```python
from build123d import *

# Parameters (mm, degrees)
SKETCH1_W           = 197
SKETCH1_H           = 107
BOSS_EXTRUDE1_DEPTH = 50
SKETCH4_W           = 182
SKETCH4_H           = 45
CUT_EXTRUDE2_DEPTH  = 25
CUT_EXTRUDE3_DEPTH  = 164
CUT_EXTRUDE12_DEPTH = 164
CUT_EXTRUDE5_DEPTH  = 230.691096911
SKETCH9_R           = 8
CUT_EXTRUDE6_DEPTH  = 171
SKETCH10_R          = 10
CUT_EXTRUDE7_DEPTH  = 1.5
SKETCH11_R          = 4.8
CUT_EXTRUDE8_DEPTH  = 12.5
SKETCH12_R          = 6.5
CUT_EXTRUDE9_DEPTH  = 230.691096911
SKETCH13_R          = 3
CUT_EXTRUDE10_DEPTH = 26.5
SKETCH14_R          = 3
CUT_EXTRUDE11_DEPTH = 26.5
CUT_EXTRUDE14_DEPTH = 35
CUT_EXTRUDE15_DEPTH = 130


with BuildPart() as part:
    # Sketch1 → Boss-Extrude1 (new body)
    with BuildSketch(Plane(origin=(0, 0, 0), x_dir=(1, 0, 0), z_dir=(0, 1, 0))):
        with Locations((98.5, 53.5)):
            Rectangle(SKETCH1_W, SKETCH1_H)
    extrude(amount=BOSS_EXTRUDE1_DEPTH)

    # Sketch4 → Cut-Extrude2 (cut)
    with BuildSketch(Plane(origin=(0, 0, 0), x_dir=(1, 0, 0), z_dir=(0, 1, 0))):
        with Locations((98.5, 53.5)):
            Rectangle(SKETCH4_W, SKETCH4_H)
    extrude(amount=CUT_EXTRUDE2_DEPTH, mode=Mode.SUBTRACT)

    # Sketch5 → Cut-Extrude3 (cut)
    with BuildSketch(Plane(origin=(197, 0, 0), x_dir=(0, 0, -1), z_dir=(1, 0, 0))):
        Polygon((58.5, 50), (107, 44.216725137), (107, 50), align=None)
    extrude(amount=-CUT_EXTRUDE3_DEPTH, mode=Mode.SUBTRACT)

    # Sketch18 → Cut-Extrude12 (cut)
    with BuildSketch(Plane(origin=(197, 0, 0), x_dir=(0, 0, -1), z_dir=(1, 0, 0))):
        Polygon((0, 44.216725137), (0, 50), (48.5, 50), align=None)
    extrude(amount=-CUT_EXTRUDE12_DEPTH, mode=Mode.SUBTRACT)

    # Sketch7 → Cut-Extrude5 (cut, through all)
    with BuildSketch(Plane(origin=(0, 0, 0), x_dir=(0, 0, -1), z_dir=(1, 0, 0))):
        Polygon((107, 50), (107, 45), (82.505102572, 50), align=None)
        Polygon((0, 45), (0, 50), (24.494897428, 50), align=None)
    extrude(amount=CUT_EXTRUDE5_DEPTH, mode=Mode.SUBTRACT)

    # Sketch9 → Cut-Extrude6 (cut)
    with BuildSketch(Plane(origin=(0, 50, 0), x_dir=(1, 0, 0), z_dir=(0, 1, 0))):
        with Locations(Location((16, 53.5, 0), (0, 0, 270))):
            Circle(SKETCH9_R)
    extrude(amount=-CUT_EXTRUDE6_DEPTH, mode=Mode.SUBTRACT)

    # Sketch10 → Cut-Extrude7 (cut)
    with BuildSketch(Plane(origin=(0, 50, 0), x_dir=(1, 0, 0), z_dir=(0, 1, 0))):
        with Locations(Location((16, 53.5, 0), (0, 0, 270))):
            Circle(SKETCH10_R)
    extrude(amount=-CUT_EXTRUDE7_DEPTH, mode=Mode.SUBTRACT)

    # Sketch11 → Cut-Extrude8 (cut)
    with BuildSketch(Plane(origin=(0, 50, 0), x_dir=(1, 0, 0), z_dir=(0, 1, 0))):
        with Locations(Location((16, 72.905102572, 0), (0, 0, 270))):
            Circle(SKETCH11_R)
        with Locations(Location((16, 34.094897428, 0), (0, 0, 270))):
            Circle(SKETCH11_R)
    extrude(amount=-CUT_EXTRUDE8_DEPTH, mode=Mode.SUBTRACT)

    # Sketch12 → Cut-Extrude9 (cut, through all)
    with BuildSketch(Plane(origin=(0, 50, 0), x_dir=(1, 0, 0), z_dir=(0, 1, 0))):
        with Locations(Location((18, 98, 0), (0, 0, 270))):
            Circle(SKETCH12_R)
        with Locations(Location((98, 9, 0), (0, 0, 270))):
            Circle(SKETCH12_R)
        with Locations(Location((178, 9, 0), (0, 0, 270))):
            Circle(SKETCH12_R)
        with Locations(Location((18, 9, 0), (0, 0, 270))):
            Circle(SKETCH12_R)
        with Locations(Location((98, 98, 0), (0, 0, 270))):
            Circle(SKETCH12_R)
        with Locations(Location((178, 98, 0), (0, 0, 270))):
            Circle(SKETCH12_R)
    extrude(amount=-CUT_EXTRUDE9_DEPTH, mode=Mode.SUBTRACT)

    # Sketch13 → Cut-Extrude10 (cut)
    with BuildSketch(Plane(origin=(0, 56.176931823, -6.698693561), x_dir=(1, 0, 0), z_dir=(0, 0.9929655081065378, -0.11840396830649387))):
        with Locations(Location((66, 88.011873646, 0), (0, 0, 270))):
            Circle(SKETCH13_R)
        with Locations(Location((158, 88.011873646, 0), (0, 0, 270))):
            Circle(SKETCH13_R)
    extrude(amount=-CUT_EXTRUDE10_DEPTH, mode=Mode.SUBTRACT)

    # Sketch14 → Cut-Extrude11 (cut)
    with BuildSketch(Plane(origin=(0, 43.2, 8.818163074), x_dir=(1, 0, 0), z_dir=(0, 0.9797958971132713, 0.2000000000000002))):
        with Locations(Location((66, 22, 0), (0, 0, 270))):
            Circle(SKETCH14_R)
        with Locations(Location((158, 22, 0), (0, 0, 270))):
            Circle(SKETCH14_R)
    extrude(amount=-CUT_EXTRUDE11_DEPTH, mode=Mode.SUBTRACT)

    # Sketch23 → Cut-Extrude14 (cut)
    with BuildSketch(Plane(origin=(0, 43.596828772, 5.198607092), x_dir=(1, 0, 0), z_dir=(0, 0.9929655081065377, 0.11840396830649416))):
        with BuildLine():
            Line((47, 49.235435722), (175, 49.235435722))
            ThreePointArc((175, 49.235435722), (178.535533906, 47.770969628), (180, 44.235435722))
            Line((180, 44.235435722), (180, 38.235435722))
            ThreePointArc((180, 38.235435722), (178.535533906, 34.699901816), (175, 33.235435722))
            Line((175, 33.235435722), (47, 33.235435722))
            ThreePointArc((47, 33.235435722), (43.464466094, 34.699901816), (42, 38.235435722))
            Line((42, 38.235435722), (42, 44.235435722))
            ThreePointArc((42, 44.235435722), (43.464466094, 47.770969628), (47, 49.235435722))
        make_face()
    extrude(amount=-CUT_EXTRUDE14_DEPTH, mode=Mode.SUBTRACT)

    # Sketch6 → Cut-Extrude15 (cut)
    with BuildSketch(Plane(origin=(0, 56.176931823, -6.698693561), x_dir=(1, 0, 0), z_dir=(0, 0.9929655081065378, -0.11840396830649387))):
        with BuildLine():
            Line((47, 73.04559264), (175, 73.04559264))
            ThreePointArc((175, 73.04559264), (178.535533906, 71.581126546), (180, 68.04559264))
            Line((180, 68.04559264), (180, 62.011873646))
            ThreePointArc((180, 62.011873646), (178.535533906, 58.47633974), (175, 57.011873646))
            Line((175, 57.011873646), (47, 57.011873646))
            ThreePointArc((47, 57.011873646), (43.464466094, 58.47633974), (42, 62.011873646))
            Line((42, 62.011873646), (42, 68.04559264))
            ThreePointArc((42, 68.04559264), (43.464466094, 71.581126546), (47, 73.04559264))
        make_face()
    extrude(amount=-CUT_EXTRUDE15_DEPTH, mode=Mode.SUBTRACT)


solid = part.part
```
Geometry check sheet. Reference: the model listing, model coordinates, mm. A direction names the side the tool comes from. Give positions to 0.01 mm unless a question says otherwise; leave off trailing zeros. Order: outer loops, then holes, each group sorted by start corner. A loop starts at its lowest first (then second) coordinate and runs counter-clockwise, first axis right, second up. Notation, with made-up numbers: (44, -24.75) - (98, -24.75) arc R31 cw to (98, 2.25) - close; hole circle Ø6 at (-10.5, -14). An arc over 180 degrees is marked (long way). Answer in a Markdown table with one row per item. Add a question column.
Q1. Cross-section at B-B, the plane x = 124. Enter the section's corners in (y, z).
Q2. Mould release check, pull along X, two halves, no side actions. Record for faces 5 (the flat face through (12.6, 48.09, -15.14)), 6 (the flat face through (7.5, 12, -53)), 7 (the flat face through (33, 48, -84)): pulls with the +X half, pulls with the -X half, needs draft (parallel to the pull), parting line crosses it, or undercut.
Q3. Cross-section at A-A, the plane z = -53.5. Enter the section's corners in (x, y), then the cut area to 3 significant figures.
Q4. Cross-section at D-D, the plane x = 98. Enter the section's corners in (y, z).
Q5. Gauge pin test, flat end, axial feed: pin 1 (21 mm diameter, centred on x = 178, z = -98, fed in from +Y). Record the tip position at first contact, or that the pin passes through.
Q6. Tool access check on faces 1 (the flat face through (16, 37.5, -34)), 2 (the cylindrical face through (95.5, 23.4, -92)), 3 (the cylindrical face through (43.426, 37.206, -43.633)), 4 (the flat face through (180, 37, -70)). Record the directions out of +Z, -Z, +X, -X, +Y, -Y that give a thin tool (end or side, any length) a straight path to the whole face; none if there is none.
Q7. Cross-section at C-C, the plane y = 6.5. Enter the section's corners in (x, z).
Q8. Material ranges on probe 1 along X at (y, z) = (11, -98); probe 2 along Z at (x, y) = (178, 23); probe 3 along Z at (x, y) = (124, 8.5), recorded low to high. Write a range as from..to.
Check values:
| question | item | result |
|---|---|---|
| 1 | outline | (0, -107) - (44.22, -107) - (47.53, -79.23) - (20.44, -76) - (0, -76) - close; (0, -31) - (20.72, -31) - (47.53, -27.8) - (44.22, 0) - (0, 0) - close; (25, -60.4) - (49.43, -63.31) - (50, -58.5) - (50, -48.5) - (49.43, -43.69) - (25, -46.6) - close |
| 2 | face 5 | needs draft |
| 2 | face 6 | undercut |
| 2 | face 7 | pulls with the +X half |
| 3 | outline | (0, 0) - (7.5, 0) - (7.5, 25) - (8, 25) - (8, 48.5) - (6, 48.5) - (6, 50) - (0, 50) - close; (24, 25) - (189.5, 25) - (189.5, 0) - (197, 0) - (197, 50) - (26, 50) - (26, 48.5) - (24, 48.5) - close |
| 3 | area | 4,890 mm^2 |
| 4 | outline | (0, -107) - (44.22, -107) - (44.51, -104.5) - (0, -104.5) - close; (0, -91.5) - (46.06, -91.5) - (47.53, -79.23) - (20.44, -76) - (0, -76) - close; (0, -31) - (20.72, -31) - (47.53, -27.8) - (46.06, -15.5) - (0, -15.5) - close; (0, -2.5) - (44.51, -2.5) - (44.22, 0) - (0, 0) - close; (25, -60.4) - (49.43, -63.31) - (50, -58.5) - (50, -48.5) - (49.43, -43.69) - (25, -46.6) - close |
| 5 | pin 1 | stops at y = 46.54 |
| 6 | face 1 | +Y |
| 6 | face 2 | +Y, -Y |
| 6 | face 3 | -Y |
| 6 | face 4 | none |
| 7 | outline | (0, -107) - (197, -107) - (197, 0) - (0, 0) - close; hole (7.5, -76) - (189.5, -76) - (189.5, -31) - (7.5, -31) - close; hole circle Ø13 at (18, -98); hole circle Ø13 at (18, -9); hole circle Ø13 at (98, -98); hole circle Ø13 at (98, -9); hole circle Ø13 at (178, -98); hole circle Ø13 at (178, -9) |
| 8 | probe 1 | x = 0..11.5, 24.5..91.5, 104.5..171.5, 184.5..197 |
| 8 | probe 2 | z = -107..-104.5, -91.5..-76, -31..-15.5, -2.5..0 |
| 8 | probe 3 | z = -107..-76, -31..0 |
